Geometry check sheet. Reference: the model listing, model coordinates, mm. Face numbers are marked on the shaded views. A direction names the side the tool comes from. Give positions to 0.01 mm unless a question says otherwise; leave off trailing zeros. Loops run counter-clockwise (first coordinate to the right, second up) from the corner with the lowest first, then second, coordinate; pieces in that order, holes last.
1. Release check for a two-part mould opening along Y. For the marked faces 1, 2, 3 and 4 record: +Y half, -Y half, draft (parallel to the pull), parting line (faces both ways), or undercut.
2. Tool access check on the marked faces 5, 6, 7 and 8. Record the directions out of +Z, -Z, +X, -X, +Y, -Y that give a thin tool (end or side, any length) a straight path to the whole face; none if there is none.
3. Cross-section at A-A, the plane y = 21. Record the cut outline in (x, z) (3 decimals), plus the area to 3 significant figures.
4. Material ranges on L1, parallel to X at y = -67.5, z = -16.5; L2, parallel to Z at x = 18.5, y = -46.75; L3, parallel to Z at x = 18.5, y = -0.8, recorded low to high.
5. Go/stop test with flat-tipped pins: pin 1 Ø12 at (y, z) = (-74, -15) entering from -X; pin 2 Ø3 at (x, y) = (21, -42) entering from +Z; pin 3 Ø4 at (y, z) = (-43.61, -16.22) entering from -X. Record where each tip stops, or that it passes through.
6. Cross-section at B-B, the plane y = -67. Record the cut outline in (x, z).
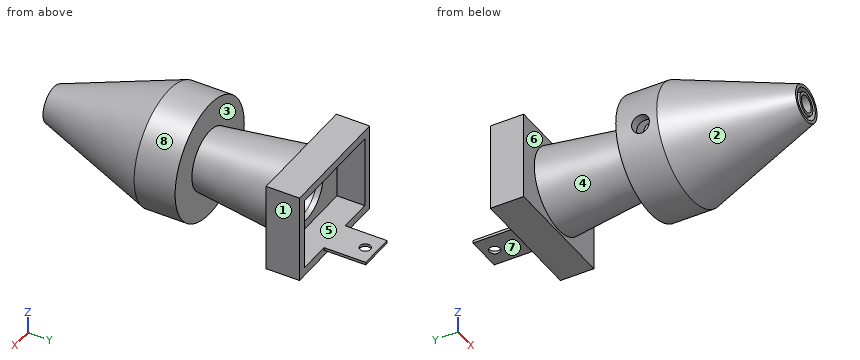
from build123d import *

# Parameters (mm, degrees)
SKETCH1_W           = 43
SKETCH1_H           = 32
SKETCH1_W_2         = 37
SKETCH1_H_2         = 26
BOSS_EXTRUDE1_DEPTH = 10
SKETCH2_W           = 13
SKETCH2_H           = 1
BOSS_EXTRUDE2_DEPTH = 15
CUT_EXTRUDE1_REACH  = 32
SKETCH3_R           = 1.905
SKETCH4_W           = 43
SKETCH4_H           = 32
BOSS_EXTRUDE3_DEPTH = 2
CUT_EXTRUDE2_REACH  = 29
SKETCH5_R           = 10
CUT_EXTRUDE3_START  = 10
SKETCH11_R          = 3.175
CUT_EXTRUDE3_DEPTH  = 15


with BuildPart() as part:
    # Sketch1 → Boss-Extrude1 (new body)
    with BuildSketch(Plane(origin=(0, 0, 0), x_dir=(1, 0, 0), z_dir=(0, 1, 0))):
        with Locations((18.5, 13)):
            Rectangle(SKETCH1_W, SKETCH1_H)
        with Locations((18.5, 13)):
            Rectangle(SKETCH1_W_2, SKETCH1_H_2, mode=Mode.SUBTRACT)
    extrude(amount=BOSS_EXTRUDE1_DEPTH)

    # Sketch2 → Boss-Extrude2 (add)
    with BuildSketch(Plane(origin=(0, 10, 0), x_dir=(1, 0, 0), z_dir=(0, 1, 0))):
        with Locations((18.5, 26.5)):
            Rectangle(SKETCH2_W, SKETCH2_H)
    extrude(amount=BOSS_EXTRUDE2_DEPTH)

    # Sketch3 → Cut-Extrude1 (cut, up to next)
    with BuildSketch(Plane(origin=(0, 0, -27), x_dir=(-1, 0, 0), z_dir=(0, 0, -1)), mode=Mode.PRIVATE) as cut_extrude1_sk1:
        with Locations((-18.5, 21)):
            Circle(SKETCH3_R)
    cut_extrude1_tool1 = extrude(cut_extrude1_sk1.sketch, amount=-CUT_EXTRUDE1_REACH, mode=Mode.PRIVATE) & part.part
    add(cut_extrude1_tool1.solids().sort_by_distance((18.5, 21, -27))[0], mode=Mode.SUBTRACT)

    # Sketch4 → Boss-Extrude3 (add)
    with BuildSketch(Plane.XZ):
        with Locations((18.5, -13)):
            Rectangle(SKETCH4_W, SKETCH4_H)
    extrude(amount=BOSS_EXTRUDE3_DEPTH)

    # Sketch5 → Cut-Extrude2 (cut, up to next)
    with BuildSketch(Plane.XZ.offset(2), mode=Mode.PRIVATE) as cut_extrude2_sk1:
        with Locations((18.5, -13)):
            Circle(SKETCH5_R)
    cut_extrude2_tool1 = extrude(cut_extrude2_sk1.sketch, amount=-CUT_EXTRUDE2_REACH, mode=Mode.PRIVATE) & part.part
    add(cut_extrude2_tool1.solids().sort_by_distance((18.5, -2, -13))[0], mode=Mode.SUBTRACT)

    # Sketch9 → Revolve1 (revolve)
    with BuildSketch(Plane.XY.offset(-13)):
        Polygon((28.5, -2), (21.5, -90.9), (22.5, -90.9), (33.5, -2), align=None)
    revolve(axis=Axis((18.5, -2, -13), (0, -1, 0)))

    # Sketch10 → Revolve2 (revolve)
    with BuildSketch(Plane.XY.offset(-13)):
        Polygon((12.988560941, -90.9), (8.633183769, -49.593045745), (0.378993359, -49.593045745), (0.378993359, -38.393027141), (8.003074224, -38.393027141), (7.567144174, -34.86991973), (-2.696890299, -34.86991973), (-2.696890299, -49.593045745), (11.935583953, -90.9), align=None)
    revolve(axis=Axis((18.5, -2, -13), (0, -1, 0)))

    # Sketch11 → Cut-Extrude3 (cut)
    with BuildSketch(Plane.ZY.offset(3).offset(CUT_EXTRUDE3_START)):
        with Locations((-16.217164304, -43.610889084)):
            Circle(SKETCH11_R)
    extrude(amount=-CUT_EXTRUDE3_DEPTH, mode=Mode.SUBTRACT)


solid = part.part
Result:
1. face 1: draft
1. face 2: -Y half
1. face 3: undercut
1. face 4: undercut
2. face 5: +Y
2. face 6: none
2. face 7: -Z, +X, -X, +Y
2. face 8: -Y
3. outline: (12, -27) - (16.595, -27) - (16.595, -26) - (12, -26) - close; (20.405, -27) - (25, -27) - (25, -26) - (20.405, -26) - close
3. area: 9.19 mm2
4. L1: x = 4.06 to 11.33, 12.56 to 15.15, 21.85 to 24.44, 25.67 to 32.94
4. L2: z = -34.2 to -31.12, -22.46 to -19.48, -6.52 to -3.54, 5.12 to 8.2
4. L3: z = -29 to -23, -3 to 3
5. pin 1: stops at x = 3.89
5. pin 2: stops at z = 8.17
5. pin 3: stops at x = 8.63
6. outline: circle Ø30.06 at (18.5, -13); circle Ø13.91 at (18.5, -13); hole circle Ø16.06 at (18.5, -13); hole circle Ø9.76 at (18.5, -13)
